Could you check a few things on this model? Use its own coordinates, in mm. Coordinates: 2 decimals unless noted, no trailing zeros. Order: outer loops, then holes, each group sorted by start corner. A loop starts at its lowest first (then second) coordinate and runs counter-clockwise, first axis right, second up. Notation, with made-up numbers: (-18, -33) -> (15, -33) arc R4 ccw to (15, -29) -> close; hole circle Ø9 at (4, 60). An arc over 180 degrees is marked (long way). Use a Markdown table: item, result. Add a question column.
1) If we section it at B-B (x = 3.5): Write out the boundary of the cut face in (y, z), plus the area to 3 significant figures.
2) If we section it at C-C (y = 31.5): Write out the boundary of the cut face in (x, z), plus the area to 3 significant figures.
3) If I drill on L1, parallel to X at y = -37, z = -1.35; L2, parallel to Y at x = -3, z = -1.3, over which ranges is the centre line in solid material (lowest first)? Write a range as [from, to].
4) Will these pins go through, and if not, where does the flat tip stop? pin 1 Ø1.2 at (x, z) = (-9, -1.5) entering from +Y; pin 2 Ø2 at (x, z) = (70, -1.5) entering from -Y.
5) If we section it at A-A (z = -2.8): Give the number of separate pieces and of enclosed holes in the cut face, plus the area to 3 significant figures.
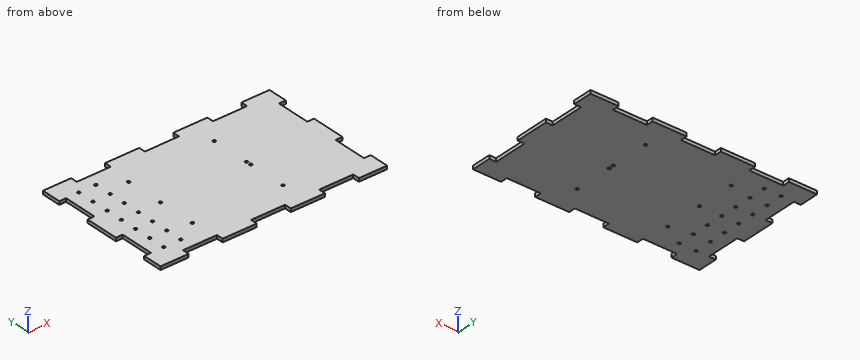
```python
from build123d import *

# Parameters (mm, degrees)
SKETCH001_W                   = 266
SKETCH001_H                   = 166
PAD_DEPTH                     = 4
SKETCH016_W                   = 30
SKETCH016_H                   = 40
SKETCH016_W_2                 = 40
SKETCH016_H_2                 = 30
POCKET001_DEPTH               = 631.146916
SKETCH016_MIRRORED002_2_W     = 30
SKETCH016_MIRRORED002_2_H     = 40
SKETCH016_MIRRORED002_2_W_2   = 40
SKETCH016_MIRRORED002_2_H_2   = 30
POCKET001_MIRRORED002_2_DEPTH = 631.146916
SKETCH035_R                   = 1.65
HOLE001_DEPTH                 = 4.001


with BuildPart() as part:
    # Sketch001 → Pad (new body)
    with BuildSketch(Plane.XY):
        Rectangle(SKETCH001_W, SKETCH001_H)
    extrude(amount=-PAD_DEPTH)

    # Sketch016 (on Face6 of Pad) → Pocket001 (cut, through all)
    with BuildSketch(Plane(origin=(0, 0, -4), x_dir=(1, 0, 0), z_dir=(0, 0, -1))):
        with Locations((140, 40)):
            Rectangle(SKETCH016_W, SKETCH016_H)
        with Locations((140, -40)):
            Rectangle(SKETCH016_W, SKETCH016_H)
        with Locations((80, -90)):
            Rectangle(SKETCH016_W_2, SKETCH016_H_2)
        with Locations((0, -90)):
            Rectangle(SKETCH016_W_2, SKETCH016_H_2)
        with Locations((-80, -90)):
            Rectangle(SKETCH016_W_2, SKETCH016_H_2)
    pocket001 = extrude(amount=-POCKET001_DEPTH, mode=Mode.SUBTRACT)

    # Sketch016 Mirrored002 2 → Pocket001 Mirrored002 2 (cut, through all)
    with BuildSketch(Plane(origin=(0, 0, -4), x_dir=(-1, 0, 0), z_dir=(0, 0, 1))):
        with Locations((140, 40)):
            Rectangle(SKETCH016_MIRRORED002_2_W, SKETCH016_MIRRORED002_2_H)
        with Locations((140, -40)):
            Rectangle(SKETCH016_MIRRORED002_2_W, SKETCH016_MIRRORED002_2_H)
        with Locations((80, -90)):
            Rectangle(SKETCH016_MIRRORED002_2_W_2, SKETCH016_MIRRORED002_2_H_2)
        with Locations((0, -90)):
            Rectangle(SKETCH016_MIRRORED002_2_W_2, SKETCH016_MIRRORED002_2_H_2)
        with Locations((-80, -90)):
            Rectangle(SKETCH016_MIRRORED002_2_W_2, SKETCH016_MIRRORED002_2_H_2)
    pocket001_mirrored002_2 = extrude(amount=POCKET001_MIRRORED002_2_DEPTH, mode=Mode.SUBTRACT)

    # Mirrored003: Pocket001, Pocket001 Mirrored002 2 across Sketch016 H_Axis
    add(pocket001.mirror(Plane(origin=(0, 0, -4), x_dir=(0, 0, -1), z_dir=(0, -1, 0))), mode=Mode.SUBTRACT)
    add(pocket001_mirrored002_2.mirror(Plane(origin=(0, 0, -4), x_dir=(0, 0, -1), z_dir=(0, -1, 0))), mode=Mode.SUBTRACT)

    # Sketch035 (on Face2 of MultiTransform) → Hole001 (cut, through all)
    with BuildSketch(Plane.XY):
        with Locations((-64, 45)):
            Circle(SKETCH035_R)
        with Locations((39.5, 48.5)):
            Circle(SKETCH035_R)
        with Locations((39.5, 3)):
            Circle(SKETCH035_R)
        with Locations((39.5, -3)):
            Circle(SKETCH035_R)
        with Locations((39.5, -48.5)):
            Circle(SKETCH035_R)
        with Locations((-64, -45)):
            Circle(SKETCH035_R)
        with Locations((-64, 0)):
            Circle(SKETCH035_R)
        with Locations((-110, -60)):
            Circle(SKETCH035_R)
        with Locations((-90, -60)):
            Circle(SKETCH035_R)
        with Locations((-110, -40)):
            Circle(SKETCH035_R)
        with Locations((-90, -40)):
            Circle(SKETCH035_R)
        with Locations((-110, -20)):
            Circle(SKETCH035_R)
        with Locations((-90, -20)):
            Circle(SKETCH035_R)
        with Locations((-110, 0)):
            Circle(SKETCH035_R)
        with Locations((-90, 0)):
            Circle(SKETCH035_R)
        with Locations((-110, 20)):
            Circle(SKETCH035_R)
        with Locations((-90, 20)):
            Circle(SKETCH035_R)
        with Locations((-110, 40)):
            Circle(SKETCH035_R)
        with Locations((-90, 40)):
            Circle(SKETCH035_R)
        with Locations((-110, 60)):
            Circle(SKETCH035_R)
        with Locations((-90, 60)):
            Circle(SKETCH035_R)
    extrude(amount=-HOLE001_DEPTH, mode=Mode.SUBTRACT)


solid = part.part
```
Answer sheet:
| question | item | result |
|---|---|---|
| 1 | outline | (-75, -4) -> (75, -4) -> (75, 0) -> (-75, 0) -> close |
| 1 | area | 600 mm2 |
| 2 | outline | (-125, -4) -> (125, -4) -> (125, 0) -> (-125, 0) -> close |
| 2 | area | 1,000 mm2 |
| 3 | L1 | [-125, 125] |
| 3 | L2 | [-75, 75] |
| 4 | pin 1 | y = 75 |
| 4 | pin 2 | y = -75 |
| 5 | separate pieces | 1 |
| 5 | enclosed holes | 21 |
| 5 | area | 40,800 mm2 |
